Build history of the part. All positions in model axes, mm. Face numbers are marked on the shaded views. A direction names the side the tool comes from. Give positions to 0.01 mm unless a question says otherwise; leave off trailing zeros. Loops run counter-clockwise (first coordinate to the right, second up) from the corner with the lowest first, then second, coordinate; pieces in that order, holes last. Notation, with made-up numbers: M 23.5,-28.5 L 38.5,-28.5 A19 ccw 38.5,5.5 Z; hole C -15.5,21 d5. An arc over 180 degrees is marked long. Put each result on its own line as item: value.
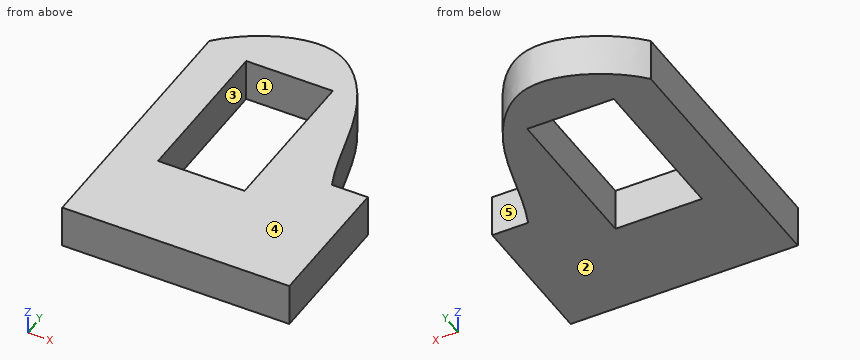
```python
from build123d import *

# Parameters (mm, degrees)
SKETCH1_W           = 64
SKETCH1_H           = 40
BOSS_EXTRUDE1_DEPTH = 12
SKETCH2_W           = 24.4
SKETCH2_H           = 45
CUT_EXTRUDE1_DEPTH  = 20


with BuildPart() as part:
    # Sketch1 → Boss-Extrude1 (new body)
    with BuildSketch(Plane.XY):
        with BuildLine():
            Line((-32, 55), (-32, 20))
            Line((-32, 20), (21.894736842, 20))
            add(Edge.make_bspline(
                [(-32, 55), (-26.093097091, 61.828307886), (-5.103314892, 73.642536114), (16.062213436, 49.100660173), (17.060908408, 31.40349279), (21.894736842, 20)],
                knots=[0, 0, 0, 0, 0.381160141, 0.579099432, 1, 1, 1, 1], degree=3))
        make_face()
        Rectangle(SKETCH1_W, SKETCH1_H)
    extrude(amount=BOSS_EXTRUDE1_DEPTH)

    # Sketch2 → Cut-Extrude1 (cut)
    with BuildSketch(Plane.XY.offset(12)):
        with Locations((-8, 30)):
            Rectangle(SKETCH2_W, SKETCH2_H)
    extrude(amount=-CUT_EXTRUDE1_DEPTH, mode=Mode.SUBTRACT)


solid = part.part
```
Q1. Slice it at B-B (x = 26). List the corners of the cut face in (y, z).
Here are the results:
outline: M -20,0 L 20,0 L 20,12 L -20,12 Z
Q2. Tool access for the marked faces 1 and 2: list every direction of +Z, -Z, +X, -X, +Y, -Y with a clear straight run to the whole face (end or side of a thin tool).
Here are the results:
face 1: +Z, -Z
face 2: -Z, +X, -X, +Y, -Y
Q3. Mould opens along Y. For the marked faces 3, 4 and 5 say: pulls with the +Y half, pulls with the -Y half, needs draft (parallel to the pull), parting line crosses it, or undercut.
Here are the results:
face 3: undercut
face 4: needs draft
face 5: pulls with the +Y half
Q4. Slice it at A-A (y = 13). List the corners of the cut face in (x, z), and give its area (3 significant figures).
Here are the results:
outline: M -32,0 L -20.2,0 L -20.2,12 L -32,12 Z; M 4.2,0 L 32,0 L 32,12 L 4.2,12 Z
area: 475 mm²
Q5. Probe line 1 (Y direction, x = 27, z = 1); line 2 (X direction, y = 13, z = 2.25); line 3 (X direction, y = 31, z = 3.75). List the from-to ranges inside material, lowest first. Write a range as from..to.
Here are the results:
line 1: -20..20
line 2: -32..-20.2, 4.2..32
line 3: -32..-20.2, 4.2..18.23
